Autodesk Inventor part; units mm, degrees
ref_plane "YZ Plane" through (0, 0, 0) normal (1, 0, 0) x (0, 1, 0)
ref_plane "XZ Plane" through (0, 0, 0) normal (0, 1, 0) x (-1, 0, 0)
ref_plane "XY Plane" through (0, 0, 0) normal (0, 0, 1) x (1, 0, 0)
sketch "Szkic1" plane through (0, 0, 0) normal (0, 1, 0) x (-1, 0, 0)
  line L0 (-28, -60) -> (29, -60)
  line L1 (-28, 60) -> (29, 60)
  line L2 (-28, 60) -> (-36, 60)
  line L3 (-36, -60) -> (-28, -60)
  circle A0 centre (-81, 0) radius 12.5
  circle A1 centre (0, 0) radius 24
  line L4 (-111, -60) -> (-36, -60)
  line L5 (-111, 60) -> (-36, 60)
  line L6 (29, 60) -> (29, -60)
  line L7 (-31, -30) -> (29, -30)
  line L8 (-31, 30) -> (29, 30)
  circle A2 centre (-81, 0) radius 15
  line L9 (-116, -60) -> (-111, -60)
  line L10 (-116, 60) -> (-111, 60)
  line L11 (-116, -60) -> (-119.57, -60)
  line L12 (-119.57, 60) -> (-116, 60)
  line L13 (-119.57, -60) -> (-122.07, -60)
  line L14 (-122.07, -60) -> (-122.07, 60)
  line L15 (-122.07, 60) -> (-119.57, 60)
  line L16 (-31, -30) -> (-31, 30)
  dimension "d0" = 30
extrude "Wyciągnięcie proste1" add sketch "Szkic1" along normal blind 8 contours L3 L4 L9 L11 L13 L14 L15 L12 L10 L5 L2 L1 L6 L8 L16 L7 L0
sketch "Szkic3" plane through (0, 8, 0) normal (0, 1, 0) x (1, 0, 0)
  line L0 (81, 15) -> (111, 15)
  line L1 (81, -15) -> (111, -15)
  arc A0 (11, -30) -> (11, 30) centre (11, 0) ccw
  circle A1 centre (81, 0) radius 15
  arc A2 (66, 15) -> (66, -15) centre (66, 0) ccw
  line L2 (81, 15) -> (66, 15)
  line L3 (81, -15) -> (66, -15)
  arc A3 (91, -15) -> (91, 15) centre (91, 0) ccw
  line L4 (116, -60) -> (116, 60)
  line L5 (111, 15) -> (116, 15)
  line L6 (111, -15) -> (116, -15)
  point P0 (0, 0)
  point P1 (116, -30)
  point P2 (116, 30)
extrude "Wyciągnięcie proste4" cut sketch "Szkic3" against normal up to next contours L0 A3 L1 A1 | A1 | A1 L3 A2 L2
sketch "Szkic4" plane through (0, 8, 0) normal (0, 1, 0) x (1, 0, 0)
  line L0 (86, -60) -> (-29, -60)
  line L1 (-29, -60) -> (-29, -30)
  line L2 (-29, -30) -> (11, -30)
  arc A0 (11, -30) -> (11, 30) centre (11, 0) ccw
  line L3 (11, 30) -> (-29, 30)
  line L4 (-29, 30) -> (-29, 60)
  line L5 (-29, 60) -> (86, 60)
  circle A1 centre (81, 0) radius 4
  circle A2 centre (0, 0) radius 5
  circle A3 centre (104.57, -23.57) radius 2.5
  circle A4 centre (57.43, -23.57) radius 2.5
  circle A5 centre (104.57, 23.57) radius 2.5
  circle A6 centre (57.43, 23.57) radius 2.5
  line L6 (122.07, 60) -> (-29, 60)
  line L7 (-29, 60) -> (-29, 30)
  line L8 (104.57, 23.57) -> (114.57, 23.57)
  line L9 (104.57, 23.57) -> (89.57, 23.57)
  arc A7 (114.57, 21.07) -> (114.57, 26.07) centre (114.57, 23.57) ccw
  arc A8 (89.57, 26.07) -> (89.57, 21.07) centre (89.57, 23.57) ccw
  line L10 (104.57, 26.07) -> (114.57, 26.07)
  line L11 (104.57, 21.07) -> (114.57, 21.07)
  line L12 (104.57, 26.07) -> (89.57, 26.07)
  line L13 (104.57, 21.07) -> (89.57, 21.07)
  circle A9 centre (104.57, -23.57) radius 2.5
  line L14 (104.57, -23.57) -> (114.57, -23.57)
  line L15 (104.57, -23.57) -> (89.57, -23.57)
  arc A10 (114.57, -26.07) -> (114.57, -21.07) centre (114.57, -23.57) ccw
  arc A11 (89.57, -21.07) -> (89.57, -26.07) centre (89.57, -23.57) ccw
  line L16 (104.57, -21.07) -> (114.57, -21.07)
  line L17 (104.57, -26.07) -> (114.57, -26.07)
  line L18 (104.57, -21.07) -> (89.57, -21.07)
  line L19 (104.57, -26.07) -> (89.57, -26.07)
  circle A12 centre (57.43, -23.57) radius 2.5
  line L20 (57.43, -23.57) -> (67.43, -23.57)
  line L21 (57.43, -23.57) -> (42.43, -23.57)
  arc A13 (67.43, -26.07) -> (67.43, -21.07) centre (67.43, -23.57) ccw
  arc A14 (42.43, -21.07) -> (42.43, -26.07) centre (42.43, -23.57) ccw
  line L22 (57.43, -21.07) -> (67.43, -21.07)
  line L23 (57.43, -26.07) -> (67.43, -26.07)
  line L24 (57.43, -21.07) -> (42.43, -21.07)
  line L25 (57.43, -26.07) -> (42.43, -26.07)
  circle A15 centre (57.43, 23.57) radius 2.5
  line L26 (57.43, 23.57) -> (67.43, 23.57)
  line L27 (57.43, 23.57) -> (42.43, 23.57)
  arc A16 (67.43, 21.07) -> (67.43, 26.07) centre (67.43, 23.57) ccw
  arc A17 (42.43, 26.07) -> (42.43, 21.07) centre (42.43, 23.57) ccw
  line L28 (57.43, 26.07) -> (67.43, 26.07)
  line L29 (57.43, 21.07) -> (67.43, 21.07)
  line L30 (57.43, 26.07) -> (42.43, 26.07)
  line L31 (57.43, 21.07) -> (42.43, 21.07)
  point P0 (0, 0)
  point P1 (86, 60)
  point P2 (116, 60)
  point P3 (119.57, 60)
  dimension "d17" = 10
  dimension "d18" = 15
  dimension "d20" = 2.5
  dimension "d22" = 10
  dimension "d23" = 15
  dimension "d24" = 2.5
  dimension "d25" = 10
  dimension "d26" = 15
  dimension "d27" = 2.5
  dimension "d28" = 10
  dimension "d29" = 15
  dimension "d30" = 2.5
extrude "Wyciągnięcie proste5" cut sketch "Szkic4" against normal up to next contours L14 L15 A3 | A3 L16 A10 L17 | A3 L15 L14 | A3 L19 A11 L18 | L20 L21 A4 | A4 L22 A13 L23 | A4 L21 L20 | A4 L25 A14 L24 | L8 L9 A5 | A5 L10 A7 L11 | A5 L9 L8 | A5 L13 A8 L12 | L26 L27 A6 | A6 L28 A16 L29 | A6 L27 L26 | A6 L31 A17 L30
fillet "Zaokrąglenie5" radius 30 2 edges at (31, 4, -30) (31, 4, 30)
fillet "Zaokrąglenie6" radius 30 2 edges at (122.07, 4, 60) (122.07, 4, -60)
sketch "Szkic5" plane through (0, 0, 0) normal (0, -1, 0) x (1, 0, 0)
  line L0 (122.07, 30) -> (122.07, -30)
  arc A0 (122.07, 30) -> (92.07, 60) centre (92.07, 30) ccw
  line L1 (-29, 60) -> (92.07, 60)
  line L2 (-29, 30) -> (-29, 60)
  arc A1 (1, -30) -> (1, 30) centre (1, 0) ccw
  line L3 (1, 30) -> (-29, 30)
  line L4 (-29, -30) -> (1, -30)
  line L5 (-29, -60) -> (-29, -30)
  line L6 (92.07, -60) -> (-29, -60)
  arc A2 (92.07, -60) -> (122.07, -30) centre (92.07, -30) ccw
  circle A3 centre (0, 0) radius 24
  arc A4 (-16.7697, 48.5) -> (-16.7697, 51.5) centre (-12, 50) ccw
  circle A5 centre (-19, 16) radius 2.5
  line L7 (-16.7697, 48.5) -> (-29, 48.5)
  line L8 (-29, 51.5) -> (-16.7697, 51.5)
  circle A6 centre (-12, -50) radius 5
  line L9 (-29, -48.5) -> (-16.7697, -48.5)
  line L10 (-16.7697, -51.5) -> (-29, -51.5)
  circle A7 centre (-19, -16) radius 2.5
  line L11 (36, -60) -> (36, 60)
  line L12 (-29, 60) -> (92.07, 60)
  line L13 (-29, 30) -> (-29, 60)
  line L14 (36, 60) -> (28, 60)
  line L15 (28, 60) -> (28, -60)
  line L16 (92.07, -60) -> (-29, -60)
  line L17 (28, -60) -> (18, -60)
  line L18 (18, -60) -> (18, 60)
  line L19 (18, -60) -> (18, -30)
  line L20 (18, 60) -> (18, 30)
  circle A8 centre (18, 30) radius 2.5
  circle A9 centre (18, -30) radius 2.5
  line L21 (18, -60) -> (3, -60)
  line L22 (3, -60) -> (3, 60)
  line L23 (3, 60) -> (3, 50)
  line L24 (3, -60) -> (3, -50)
  circle A10 centre (3, 50) radius 2.5
  circle A11 centre (3, -50) radius 2.5
  line L25 (28, -60) -> (23, -60)
  line L26 (92.07, -60) -> (-29, -60)
  line L27 (23, -60) -> (23, 60)
  line L28 (-29, 60) -> (92.07, 60)
  circle A12 centre (23, 30) radius 2.5
  circle A13 centre (23, -30) radius 2.5
  point P0 (0, 0)
  dimension "d36" = 8
  dimension "d37" = 10
  dimension "d38" = 30
  dimension "d39" = 30
  dimension "d40" = 5
  dimension "d41" = 5
  dimension "d42" = 15
  dimension "d43" = 10
  dimension "d44" = 10
  dimension "d45" = 5
  dimension "d46" = 5
  dimension "d49" = 5
  dimension "d50" = 5
  dimension "d51" = 5
extrude "Wyciągnięcie proste7" cut sketch "Szkic5" against normal up to next contours A12 L27 | L27 A12 | A13 L27 | L27 A13 | A10 L22 | L22 A10 | A11 L22 | L22 A11
properties part number "Uchwyt silnika krokowego osi Zi"
Design review of the part built by this model. Coordinates are the model's own, in mm. A direction names the side the tool comes from. Coordinates: 2 decimals unless noted, no trailing zeros. Write each loop counter-clockwise with the first axis right and the second up, starting at its lowest first coordinate (ties: lowest second). Pieces come first, ordered by that corner, then holes. Notation, with made-up numbers: M -18,54 L 23,54 A23 cw 23,88 Z; hole C 26,18 d8. An arc over 180 degrees is marked long. Answer as a JSON object with one key per item and string values.
Item 1: Add section C-C, the plane z = -23.57. Give the boundary of the cut face in (x, y), and give its area (3 significant figures).
Outcome:
{"outline": "M 19.56,0 L 39.93,0 L 39.93,8 L 19.56,8 Z; M 69.93,0 L 87.07,0 L 87.07,8 L 69.93,8 Z; M 117.07,0 L 122.07,0 L 122.07,8 L 117.07,8 Z", "area": "340 mm²"}
Item 2: Machinability: for faces 5 (the cylindrical face through (51, 4, 0)), 6 (the flat face through (122.07, 4, 0)), which of the approach directions +Z, -Z, +X, -X, +Y, -Y give a long, thin tool a straight path to every point of the face, cutting with its end or side? Answer none if there is none.
Outcome:
{"face 5": "+Y, -Y", "face 6": "+Z, -Z, +X, +Y, -Y"}
Item 3: Insertion check: pin 1 Ø1.5 at (x, y) = (96.5, 4) entering from -Z; pin 2 Ø1.5 at (y, z) = (2.5, -11) entering from -X. Each pin has a flat end and moves straight along its axis. Give the tip position at first contact, or say it passes through.
Outcome:
{"pin 1": "z = -59.77", "pin 2": "x = 28.6"}
Item 4: Draft analysis for pull direction X (two halves, no side actions). For faces 1 (the cylindrical face through (106, 4, 0)), 2 (the cylindrical face through (113.049, 4.056, 51.445)), 3 (the flat face through (-14, 4, 30)), 4 (the cylindrical face through (87.07, 4.06, 23.52)), state which applies: pulls with the +X half, pulls with the -X half, needs draft (parallel to the pull), parting line crosses it, or undercut.
Outcome:
{"face 1": "undercut", "face 2": "pulls with the +X half", "face 3": "needs draft", "face 4": "undercut"}
Item 5: Wall thickness on probe 1 along Z at (x, y) = (23, 1.5); probe 2 along Z at (x, y) = (115.5, 2.5); probe 3 along Z at (x, y) = (3, 2): over which ranges is each line inside the solid? List them lowest first.
Outcome:
{"probe 1": "-60 to -32.5, -27.5 to -20.4, 20.4 to 27.5, 32.5 to 60", "probe 2": "-48.74 to -25.89, -21.25 to 21.25, 25.89 to 48.74", "probe 3": "-60 to -52.5, -47.5 to -29.93, 29.93 to 47.5, 52.5 to 60"}
Item 6: Add section D-D, the plane z = -6. Give the boundary of the cut face in (x, y).
Outcome:
{"outline": "M 30.39,0 L 52.25,0 L 52.25,8 L 30.39,8 Z; M 104.75,0 L 122.07,0 L 122.07,8 L 104.75,8 Z"}
Item 7: Add section B-B, the plane x = -7. Give the boundary of the cut face in (y, z).
Outcome:
{"outline": "M 0,-60 L 8,-60 L 8,-30 L 0,-30 Z; M 0,30 L 8,30 L 8,60 L 0,60 Z"}
Item 8: Add section A-A, the plane x = 48.5. Give the boundary of the cut face in (y, z).
Outcome:
{"outline": "M 0,-60 L 8,-60 L 8,-26.07 L 0,-26.07 Z; M 0,-21.07 L 8,-21.07 L 8,21.07 L 0,21.07 Z; M 0,26.07 L 8,26.07 L 8,60 L 0,60 Z"}
